from build123d import *

# Parameters (mm, degrees)
EXTRUDE_1_DEPTH          = 16
CUT_EXTRUDE_1_DEPTH      = 256.501467706
CUT_EXTRUDE_1_DEPTH_BACK = 256.501467706
SKETCH_2_R               = 9
CUT_EXTRUDE_2_DEPTH      = 256.501467706
CUT_EXTRUDE_2_DEPTH_BACK = 256.501467706
SKETCH_3_R               = 6
CUT_EXTRUDE_3_DEPTH      = 256.501467706
CUT_EXTRUDE_3_DEPTH_BACK = 256.501467706
SKETCH_4_R               = 5.053


with BuildPart() as part:
    # ｽｹｯﾁ1 → ﾎﾞｽ - 押し出し1 (new body)
    with BuildSketch(Plane(origin=(0, 0, 0), x_dir=(1, 0, 0), z_dir=(0, 1, 0))):
        with BuildLine():
            Line((-215, -120), (65, -120))
            Line((65, -120), (75, -110))
            Line((75, -110), (75, -70))
            ThreePointArc((75, -70), (77.928932188, -62.928932188), (85, -60))
            Line((85, -60), (225, -60))
            Line((225, -60), (225, 60))
            Line((225, 60), (85, 60))
            ThreePointArc((85, 60), (77.928932188, 62.928932188), (75, 70))
            Line((75, 70), (75, 110))
            Line((75, 110), (65, 120))
            Line((65, 120), (-215, 120))
            Line((-215, 120), (-225, 110))
            Line((-225, 110), (-225, -110))
            Line((-225, -110), (-215, -120))
        make_face()
    extrude(amount=EXTRUDE_1_DEPTH)

    # ｽｹｯﾁ2 → ｶｯﾄ - 押し出し1 (cut, two sides: drawn at the far end of the back side and taken through both)
    with BuildSketch(Plane(origin=(0, 0, 0), x_dir=(1, 0, 0), z_dir=(0, 1, 0)).offset(-CUT_EXTRUDE_1_DEPTH_BACK)):
        with Locations(Location((-75, -95, 0), (0, 0, 270))):
            Circle(SKETCH_2_R)
        with Locations(Location((-75, 95, 0), (0, 0, 270))):
            Circle(SKETCH_2_R)
    extrude(amount=CUT_EXTRUDE_1_DEPTH + CUT_EXTRUDE_1_DEPTH_BACK, mode=Mode.SUBTRACT)

    # ｽｹｯﾁ3 → ｶｯﾄ - 押し出し2 (cut, two sides: drawn at the far end of the back side and taken through both)
    with BuildSketch(Plane(origin=(0, 0, 0), x_dir=(1, 0, 0), z_dir=(0, 1, 0)).offset(-CUT_EXTRUDE_2_DEPTH_BACK)):
        with Locations(Location((-185, -40, 0), (0, 0, 270))):
            Circle(SKETCH_3_R)
        with Locations(Location((-185, 40, 0), (0, 0, 270))):
            Circle(SKETCH_3_R)
        with Locations(Location((185, -40, 0), (0, 0, 270))):
            Circle(SKETCH_3_R)
        with Locations(Location((185, 40, 0), (0, 0, 270))):
            Circle(SKETCH_3_R)
    extrude(amount=CUT_EXTRUDE_2_DEPTH + CUT_EXTRUDE_2_DEPTH_BACK, mode=Mode.SUBTRACT)

    # ｽｹｯﾁ4 → ｶｯﾄ - 押し出し3 (cut, two sides: drawn at the far end of the back side and taken through both)
    with BuildSketch(Plane(origin=(0, 0, 0), x_dir=(1, 0, 0), z_dir=(0, 1, 0)).offset(-CUT_EXTRUDE_3_DEPTH_BACK)):
        with Locations(Location((-205, -40, 0), (0, 0, 270))):
            Circle(SKETCH_4_R)
        with Locations(Location((-205, 40, 0), (0, 0, 270))):
            Circle(SKETCH_4_R)
        with Locations(Location((0, -40, 0), (0, 0, 270))):
            Circle(SKETCH_4_R)
        with Locations(Location((0, 40, 0), (0, 0, 270))):
            Circle(SKETCH_4_R)
        with Locations(Location((205, -40, 0), (0, 0, 270))):
            Circle(SKETCH_4_R)
        with Locations(Location((205, 40, 0), (0, 0, 270))):
            Circle(SKETCH_4_R)
    extrude(amount=CUT_EXTRUDE_3_DEPTH + CUT_EXTRUDE_3_DEPTH_BACK, mode=Mode.SUBTRACT)


solid = part.part
Verification items for the finished model (mm, model axes). A direction names the side the tool comes from. Coordinates: 2 decimals unless noted, no trailing zeros. Write each loop counter-clockwise with the first axis right and the second up, starting at its lowest first coordinate (ties: lowest second). Pieces come first, ordered by that corner, then holes. Notation, with made-up numbers: (36, 76) -> (80, 76) arc R27 ccw to (80, 115) -> close; hole circle Ø3 at (-7, 82). An arc over 180 degrees is marked (long way). One line per item, written item: value. Start each with the question number.
Q1. Access from +Z, -Z, +X, -X, +Y, -Y to the whole of each face (thin tool, end or side, straight path). Record for faces 1 (the flat face through (-73, 8, -120)), 2 (the flat face through (75, 8, -90)), 3 (the flat face through (154, 8, 60)).
Q2. Thickness scan on L1, parallel to X at y = 4.75, z = -40; L2, parallel to Z at x = 205, y = 5.25; L3, parallel to Z at x = -185, y = 9. Record the ranges inside material, lowest first. Write a range as from..to.
Q3. Cross-section at C-C on y = 9. State how many separate pieces and enclosed holes the cut face has, and give its area (3 significant figures).
Q4. Cross-section at D-D on z = -40. Enter the section's corners in (x, y).
Q5. Go/stop test with flat-tipped pins: P1, Ø5, axis at x = 179.5, y = 10.5, coming from the -Z side; P2, Ø8, axis at y = 4, z = 95.5, coming from the +X side; P3, Ø16, axis at x = -75, z = 95, coming from the -Y side; P4, Ø5, axis at x = 160.5, y = 5.5, coming from the +Z side. Record where each tip stops, or that it passes through.
Q6. Mould release check, pull along X, two halves, no side actions. Record for faces 4 (the flat face through (70, 8, 115)), 5 (the flat face through (-53, 0, -2)), 6 (the cylindrical face through (200.07, 7.89, -41.1)): pulls with the +X half, pulls with the -X half, needs draft (parallel to the pull), parting line crosses it, or undercut.
Q7. Cross-section at B-B on z = -95. Enter the section's corners in (x, y), and give its area (3 significant figures).
Q8. Cross-section at A-A on x = 185. Enter the section's corners in (y, z).
Checked values:
1. face 1: -Z, +X, -X, +Y, -Y
1. face 2: -Z, +X, +Y, -Y
1. face 3: +Z, +X, +Y, -Y
2. L1: x = -225..-210.05, -199.95..-191, -179..-5.05, 5.05..179, 191..199.95, 210.05..225
2. L2: z = -60..-45.05, -34.95..34.95, 45.05..60
2. L3: z = -120..-46, -34..34, 46..120
3. separate pieces: 1
3. enclosed holes: 12
3. area: 88,400 mm²
4. outline: (-225, 0) -> (-210.05, 0) -> (-210.05, 16) -> (-225, 16) -> close; (-199.95, 0) -> (-191, 0) -> (-191, 16) -> (-199.95, 16) -> close; (-179, 0) -> (-5.05, 0) -> (-5.05, 16) -> (-179, 16) -> close; (5.05, 0) -> (179, 0) -> (179, 16) -> (5.05, 16) -> close; (191, 0) -> (199.95, 0) -> (199.95, 16) -> (191, 16) -> close; (210.05, 0) -> (225, 0) -> (225, 16) -> (210.05, 16) -> close
5. P1: stops at z = -60
5. P2: stops at x = 75
5. P3: passes through
5. P4: stops at z = 60
6. face 4: pulls with the +X half
6. face 5: needs draft
6. face 6: undercut
7. outline: (-225, 0) -> (-84, 0) -> (-84, 16) -> (-225, 16) -> close; (-66, 0) -> (75, 0) -> (75, 16) -> (-66, 16) -> close
7. area: 4,510 mm²
8. outline: (0, -60) -> (16, -60) -> (16, -46) -> (0, -46) -> close; (0, -34) -> (16, -34) -> (16, 34) -> (0, 34) -> close; (0, 46) -> (16, 46) -> (16, 60) -> (0, 60) -> close
